For this review, take the finished solid that the model builds, in its own axes (mm). A direction names the side the tool comes from. Round coordinates to 2 decimals unless told otherwise and drop trailing zeros. Loops run counter-clockwise (first coordinate to the right, second up) from the corner with the lowest first, then second, coordinate; pieces in that order, holes last.
1. Tool access review of faces 1 (the cylindrical face through (-141.96, 51.993, 195.996)), 2 (the cylindrical face through (-18.241, 55.487, 170.485)): name each direction out of +Z, -Z, +X, -X, +Y, -Y from which nothing blocks a thin tool from reaching the whole face with its end or side.
2. To check wall thickness, follow line 1 along Y through (x, z) = (-23, 180.5); line 2 along Z through (x, y) = (-17, 47); line 3 along Z through (x, y) = (-143, 52). State the ranges of each line that lie inside material, in increasing order.
3. Consider section B-B on x = -206. State the section outline as (y, z) points, then the cut area to 3 significant figures.
4. Clearance check with flat-ended pins moving along their axes: pin 1 Ø10.5 at (y, z) = (48.5, 178) entering from +X; pin 2 Ø10 at (x, y) = (-213.5, 44) entering from +Z; pin 3 Ø6 at (x, y) = (-78, 64.5) entering from -Z. State where each tip first meets the part, or that it passes through.
5. Consider section A-A on y = 45. State the section outline as (x, z) points, then the cut area to 3 significant figures.
from build123d import *

# Parameters (mm, degrees)
SKETCH3_W               = 280
SKETCH3_H               = 31
BOSS_EXTRUDE1_DEPTH     = 196
CUT_EXTRUDE1_DEPTH      = 349.449961347
CUT_EXTRUDE1_DEPTH_BACK = 349.449961347
SKETCH6_R               = 10.5
CUT_EXTRUDE2_DEPTH      = 37


with BuildPart() as part:
    # Sketch3 → Boss-Extrude1 (new body)
    with BuildSketch(Plane.XY):
        with Locations((-140, 52.333439857)):
            Rectangle(SKETCH3_W, SKETCH3_H)
    extrude(amount=BOSS_EXTRUDE1_DEPTH)

    # Sketch4 → Cut-Extrude1 (cut, two sides: drawn at the far end of the back side and taken through both)
    with BuildSketch(Plane(origin=(0, 0, 0), x_dir=(0, 0, -1), z_dir=(1, 0, 0)).offset(-CUT_EXTRUDE1_DEPTH_BACK)):
        with BuildLine():
            Line((-180.5, 67.833439857), (-180.5, 68.833439857))
            Line((-180.5, 68.833439857), (-197, 68.833439857))
            Line((-197, 68.833439857), (-197, 35.833439857))
            Line((-197, 35.833439857), (-180.5, 35.833439857))
            Line((-180.5, 35.833439857), (-180.5, 36.833439857))
            ThreePointArc((-180.5, 36.833439857), (-196, 52.333439857), (-180.5, 67.833439857))
        make_face()
        with BuildLine():
            Line((-15.5, 67.833439857), (-15.5, 68.833439857))
            Line((-15.5, 68.833439857), (1, 68.833439857))
            Line((1, 68.833439857), (1, 35.833439857))
            Line((1, 35.833439857), (-15.5, 35.833439857))
            Line((-15.5, 35.833439857), (-15.5, 36.833439857))
            ThreePointArc((-15.5, 36.833439857), (0, 52.333439857), (-15.5, 67.833439857))
        make_face()
    extrude(amount=CUT_EXTRUDE1_DEPTH + CUT_EXTRUDE1_DEPTH_BACK, mode=Mode.SUBTRACT)

    # Sketch6 → Cut-Extrude2 (cut)
    with BuildSketch(Plane(origin=(0, 0, 0), x_dir=(0, 0, -1), z_dir=(1, 0, 0))):
        with Locations((-180.5, 52.333439857)):
            Circle(SKETCH6_R)
        with Locations((-15.5, 52.333439857)):
            Circle(SKETCH6_R)
    extrude(amount=-CUT_EXTRUDE2_DEPTH, mode=Mode.SUBTRACT)


solid = part.part
Resolved:
1. face 1: +Z, +X, -X
1. face 2: +X
2. line 1: y = 36.83 to 41.83, 62.83 to 67.83
2. line 2: z = 0.95 to 6.46, 24.54 to 171.46, 189.54 to 195.05
2. line 3: z = 0 to 196
3. outline: (36.83, 15.5) arc R15.5 ccw to (67.83, 15.5) - (67.83, 180.5) arc R15.5 ccw to (36.83, 180.5) - close
3. area: 5,870 mm2
4. pin 1: stops at x = -37
4. pin 2: stops at z = 195.64
4. pin 3: stops at z = 3
5. outline: (-280, 1.84) - (0, 1.84) - (0, 7.99) - (-37, 7.99) - (-37, 23.01) - (0, 23.01) - (0, 172.99) - (-37, 172.99) - (-37, 188.01) - (0, 188.01) - (0, 194.16) - (-280, 194.16) - close
5. area: 52,700 mm2
